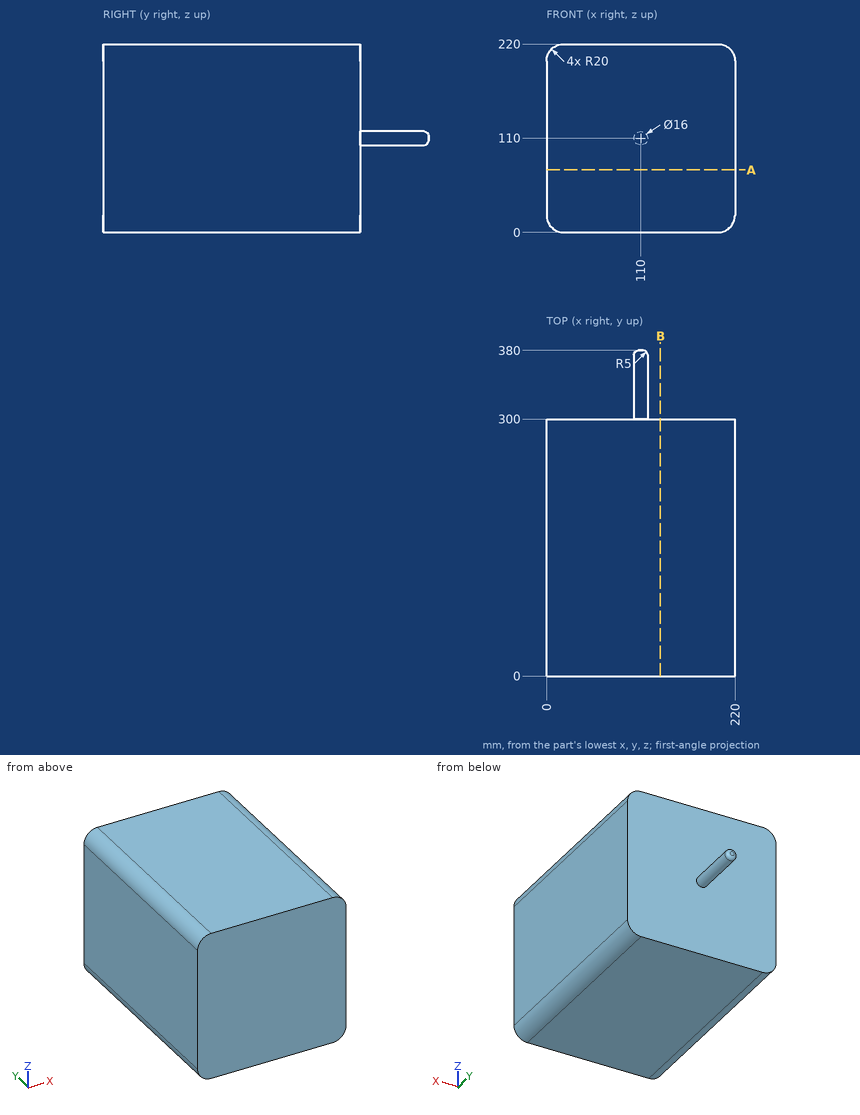
Part print with two shaded views. Sizes in mm from the minimum x, y, z corner. Give positions to 0.01 mm unless a question says otherwise; leave off trailing zeros. Order: outer loops, then holes, each group sorted by start corner. A loop starts at its lowest first (then second) coordinate and runs counter-clockwise, first axis right, second up.
(1) Saw through at A-A, the plane z = 73. Give the cut face in (x, y).
(2) Flat gauge pins, fed straight in: pin 1 (10 mm diameter, centred on x = 29, z = 69.5, fed in from +Y); pin 2 (1.5 mm diameter, centred on x = 102.5, z = 31, fed in from -Y). Where does each tip first touch, or does it go through?
(3) Saw through at B-B, the plane x = 133. Give the cut face in (y, z).
(4) Drill centre lines: L1, parallel to Y at x = 83, z = 119.5; L2, parallel to Z at x = 15, y = 258; L3, parallel to Z at x = 12, y = 233.5. Where is each one in solid material? Low to high.
Results found:
1. outline: (0, 0) - (220, 0) - (220, 300) - (0, 300) - close
2. pin 1: stops at y = 300
2. pin 2: stops at y = 0
3. outline: (0, 0) - (300, 0) - (300, 220) - (0, 220) - close
4. L1: y = 0 to 300
4. L2: z = 0.64 to 219.36
4. L3: z = 1.67 to 218.33
